Source: CAD feature listing. Evaluate the final solid. Frame: model axes, mm. Coordinates: 2 decimals unless noted, no trailing zeros. Loops run counter-clockwise (first coordinate to the right, second up) from the corner with the lowest first, then second, coordinate; pieces in that order, holes last.
Item 1: Line query: probe 1 along Y at (x, z) = (-84, 1.5); probe 2 along X at (y, z) = (101, 2.4); probe 3 along X at (y, z) = (24, 4.3). Output: solid intervals per line, ascending.
Item 2: Section query A-A, the plane y = 85. Return the cut outline in (x, z), then the cut area to 3 significant figures.
Item 3: Pull-direction query (Y, two-part tool) for faces 1 (the flat face through (-54, 110, 2)), 2 (the cylindrical face through (-2.255, 2.139, 2.535)), 3 (the cylindrical face through (-8.49, 83.09, 2.47)); classes: +Y half, -Y half, draft (parallel to the pull), parting line (faces both ways), or undercut.
```python
from build123d import *

# Parameters (mm, degrees)
SKETCH_1_W         = 110
SKETCH_1_H         = 110
EXTRUDE_1_DEPTH    = 5
HOLE_WIZARD_M2_1_D = 2.4
HOLE_WIZARD_M4_1_D = 4.3
FILLET_1_R         = 7.5


with BuildPart() as part:
    # ｽｹｯﾁ1 → ﾎﾞｽ - 押し出し1 (new body)
    with BuildSketch(Plane(origin=(0, 0, 0), x_dir=(0, 1, 0), z_dir=(0, 0, 1))):
        with Locations((55, 55)):
            Rectangle(SKETCH_1_W, SKETCH_1_H)
    extrude(amount=EXTRUDE_1_DEPTH)

    # M2 すきま穴1 (through all)
    with Locations(Plane.XY.offset(5)):
        with Locations((-84, 9), (-84, 101), (-26, 101), (-26, 9)):
            Hole(HOLE_WIZARD_M2_1_D / 2)

    # M4 すきま穴1 (through all)
    with Locations(Plane.XY.offset(5)):
        with Locations((-102.5, 85), (-102.5, 25), (-7.5, 25), (-7.5, 85)):
            Hole(HOLE_WIZARD_M4_1_D / 2)

    # ﾌｨﾚｯﾄ1
    fillet_1_edges = [part.edges().sort_by_distance(p)[0] for p in [
        (-110, 0, 2.5),
        (-110, 110, 2.5),
        (0, 110, 2.5),
        (0, 0, 2.5),
    ]]
    fillet(fillet_1_edges, radius=FILLET_1_R)


solid = part.part
```
Verdict:
1. probe 1: y = 0 to 7.8, 10.2 to 99.8, 102.2 to 110
1. probe 2: x = -110 to -85.2, -82.8 to -27.2, -24.8 to 0
1. probe 3: x = -110 to -104.4, -100.6 to -9.4, -5.6 to 0
2. outline: (-110, 0) - (-104.65, 0) - (-104.65, 5) - (-110, 5) - close; (-100.35, 0) - (-9.65, 0) - (-9.65, 5) - (-100.35, 5) - close; (-5.35, 0) - (0, 0) - (0, 5) - (-5.35, 5) - close
2. area: 507 mm2
3. face 1: +Y half
3. face 2: -Y half
3. face 3: undercut
